Check sheet for the modelled part. Datum: model origin and axes. Units: mm. Face numbers are marked on the shaded views. A direction names the side the tool comes from. Give positions to 0.01 mm unless a question says otherwise; leave off trailing zeros. Loops run counter-clockwise (first coordinate to the right, second up) from the corner with the lowest first, then second, coordinate; pieces in that order, holes last. Notation, with made-up numbers: M 4.5,21.5 L 60.5,21.5 A13 ccw 60.5,33.5 Z; hole C -12,18 d10. An arc over 180 degrees is marked long. Put each result on its own line as item: value. Start each with the question number.
Autodesk Inventor part; units mm, degrees
ref_plane "YZ Plane" through (0, 0, 0) normal (1, 0, 0) x (0, 1, 0)
ref_plane "XZ Plane" through (0, 0, 0) normal (0, 1, 0) x (-1, 0, 0)
ref_plane "XY Plane" through (0, 0, 0) normal (0, 0, 1) x (1, 0, 0)
sketch "Sketch1" plane through (0, 0, 0) normal (0, 0, 1) x (1, 0, 0)
  circle A0 centre (0, 0) radius 14.25
  dimension "d0" = 28.5
extrude "Extrusion1" add sketch "Sketch1" along normal blind 125
sketch "Sketch2" plane through (0, 0, 125) normal (0, 0, 1) x (1, 0, 0)
  circle A0 centre (0, 0) radius 7.9375
  dimension "d3" = 15.875
extrude "Extrusion2" add sketch "Sketch2" along normal blind 12.5
sketch "Sketch3" plane through (0, 0, 137.5) normal (0, 0, 1) x (1, 0, 0)
  circle A0 centre (0, 0) radius 4
  dimension "d6" = 8
extrude "Extrusion3" cut sketch "Sketch3" against normal blind 50.8
sketch "Sketch4" plane through (0, 0, 0) normal (0, 0, -1) x (-1, 0, 0)
  circle A0 centre (0, 0) radius 7.9375
  dimension "d9" = 15.875
extrude "Extrusion4" add sketch "Sketch4" along normal blind 16
sketch "Sketch5" plane through (0, 0, -16) normal (0, 0, -1) x (-1, 0, 0)
  line L0 (-4.75, -7.9375) -> (4.75, -7.9375)
  line L1 (4.75, -7.9375) -> (4.75, 7.9375)
  line L2 (4.75, 7.9375) -> (-4.75, 7.9375)
  line L3 (-4.75, 7.9375) -> (-4.75, -7.9375)
  line L4 (-4.75, -7.9375) -> (4.75, 7.9375) construction
  line L5 (4.75, -7.9375) -> (-4.75, 7.9375) construction
  circle A0 centre (0, 0) radius 7.9375 construction
  circle A1 centre (0, 0) radius 7.9375
  arc A2 (-4.8155, 6.3099) -> (-4.8155, -6.3099) centre (0, 0) ccw
  arc A3 (4.7611, -6.351) -> (4.7611, 6.351) centre (0, 0) ccw
  line L6 (-4.8155, 6.3099) -> (-4.8155, -6.3099)
  line L7 (4.7611, 6.351) -> (4.7611, -6.351)
  dimension "d12" = 9.5
extrude "Extrusion5" cut sketch "Sketch5" against normal up to surface (16 mm away) contours A1 L6 | L7 A1
sketch "Sketch6" plane through (4.8155, -6.3099, -16) normal (1, 0, 0) x (0, 0, -1)
  line L0 (0, -0.0411) -> (0, 12.6609) construction
  line L1 (0, 6.3099) -> (-7, 6.3099) construction
  circle A0 centre (-7, 6.3099) radius 3.2
  point P0 (-16, 6.3099)
  dimension "d15" = 6.4
  dimension "d16" = 7
extrude "Extrusion6" cut sketch "Sketch6" against normal through all
properties part number "cylinder"
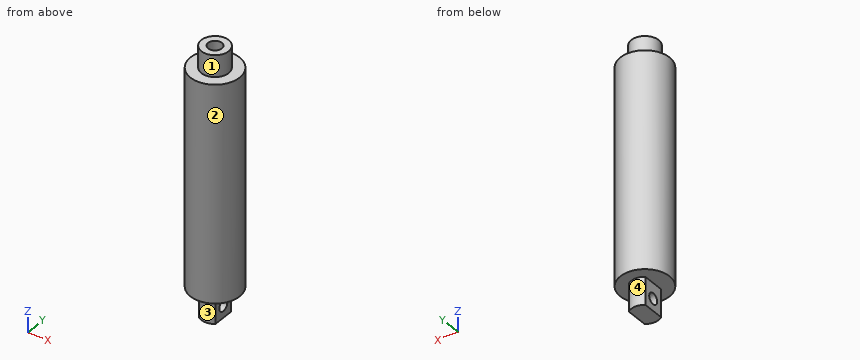
Q1. Section check C-C, the plane z = -9. Record the cut outline in (x, y) (1 decimal).
Q2. Section check D-D, the plane z = 117. Record the cut outline in (x, y).
Q3. Thickness scan on line 1 along Y through (x, z) = (-0.25, -9); line 2 along Y through (x, z) = (0, 103); line 3 along Z through (x, y) = (7.25, -10.25). Record the ranges inside material, lowest first. Write a range as [from, to].
Q4. Section check B-B, the plane x = 0. Record the cut outline in (y, z).
Q5. Access from +Z, -Z, +X, -X, +Y, -Y to the whole of each face (thin tool, end or side, straight path). Record for the marked faces 1, 2, 3 and 4.
Q6. Section check A-A, the plane y = 0. Record the cut outline in (x, z).
Q7. Depth check by flat-ended pin: P1, Ø4, axis at x = -7, z = 3, coming from the -Y side; P2, Ø7.5, axis at y = 0, z = -9, coming from the -X side; P3, Ø4, axis at y = 1, z = -10.5, coming from the +X side. Enter the tip coordinate at first touch or a pass-through.
Found:
1. outline: M -4.8,-6.4 A7.9 ccw 4.8,-6.3 L 4.8,-3.2 L -4.8,-3.2 Z; M -4.8,3.2 L 4.8,3.2 L 4.8,6.3 A7.9 ccw -4.8,6.4 Z
2. outline: C 0,0 d28.5; hole C 0,0 d8
3. line 1: y = [-7.93, -3.2], [3.2, 7.93]
3. line 2: y = [-14.25, -4], [4, 14.25]
3. line 3: z = [0, 125]
4. outline: M -14.25,0 L -7.94,0 L -7.94,-16 L 7.94,-16 L 7.94,0 L 14.25,0 L 14.25,125 L 7.94,125 L 7.94,137.5 L 4,137.5 L 4,86.7 L -4,86.7 L -4,137.5 L -7.94,137.5 L -7.94,125 L -14.25,125 Z; hole C 0,-9 d6.4
5. face 1: +Z
5. face 2: +Z, -Z
5. face 3: -Z, -Y
5. face 4: -Z, +Y
6. outline: M -14.25,0 L -4.76,0 L -4.76,-5.8 L 4.82,-5.8 L 4.82,0 L 14.25,0 L 14.25,125 L 7.94,125 L 7.94,137.5 L 4,137.5 L 4,86.7 L -4,86.7 L -4,137.5 L -7.94,137.5 L -7.94,125 L -14.25,125 Z; M -4.76,-16 L 4.82,-16 L 4.82,-12.2 L -4.76,-12.2 Z
7. P1: stops at y = -13.34
7. P2: stops at x = -4.76
7. P3: stops at x = 4.82
